Here's how the part is built. I have some questions about the finished solid (model axes, mm). Face numbers are marked on the shaded views. Coordinates: 2 decimals unless noted, no trailing zeros. Write each loop counter-clockwise with the first axis right and the second up, starting at its lowest first coordinate (ties: lowest second). Pieces come first, ordered by that corner, then holes.
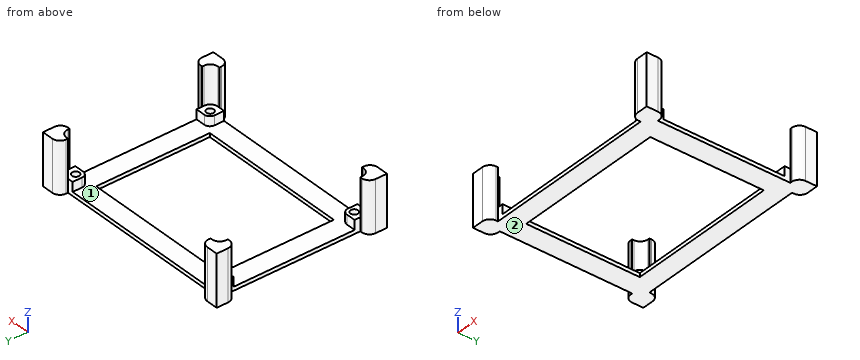
```python
from build123d import *

# Parameters (mm, degrees)
BOSS_EXTRUDE2_DEPTH = 27
SKETCH3_W           = 102
SKETCH3_H           = 80
CUT_EXTRUDE2_DEPTH  = 25
SKETCH4_W           = 8
SKETCH4_H           = 8
BOSS_EXTRUDE3_DEPTH = 5
SKETCH7_R           = 1.95
CUT_EXTRUDE3_DEPTH  = 3
FILLET2_R           = 3
FILLET3_R           = 4
SKETCH8_W           = 80
SKETCH8_H           = 60
CUT_EXTRUDE4_DEPTH  = 3


with BuildPart() as part:
    # Sketch1 → Boss-Extrude2 (new body)
    with BuildSketch(Plane.XY):
        Polygon((0, 75), (-5, 75), (-5, 85), (5, 85), (5, 80), (97, 80), (97, 85), (107, 85), (107, 75), (102, 75), (102, 5), (107, 5), (107, -5), (97, -5), (97, 0), (5, 0), (5, -5), (-5, -5), (-5, 5), (0, 5), align=None)
    extrude(amount=BOSS_EXTRUDE2_DEPTH)

    # Sketch3 → Cut-Extrude2 (cut)
    with BuildSketch(Plane.XY.offset(27)):
        with Locations((51, 40)):
            Rectangle(SKETCH3_W, SKETCH3_H)
    extrude(amount=-CUT_EXTRUDE2_DEPTH, mode=Mode.SUBTRACT)

    # Sketch4 → Boss-Extrude3 (add)
    with BuildSketch(Plane.XY.offset(2)):
        with Locations((4, 76)):
            Rectangle(SKETCH4_W, SKETCH4_H)
        with Locations((98, 76)):
            Rectangle(SKETCH4_W, SKETCH4_H)
        with Locations((98, 4)):
            Rectangle(SKETCH4_W, SKETCH4_H)
        with Locations((4, 4)):
            Rectangle(SKETCH4_W, SKETCH4_H)
    extrude(amount=BOSS_EXTRUDE3_DEPTH)

    # Sketch7 → Cut-Extrude3 (cut)
    with BuildSketch(Plane.XY.offset(7)):
        with Locations((4.5, 75.5)):
            Circle(SKETCH7_R)
        with Locations((97.5, 75.5)):
            Circle(SKETCH7_R)
        with Locations((97.5, 4.5)):
            Circle(SKETCH7_R)
        with Locations((4.5, 4.5)):
            Circle(SKETCH7_R)
    extrude(amount=-CUT_EXTRUDE3_DEPTH, mode=Mode.SUBTRACT)

    # Fillet2
    fillet2_edges = [part.edges().sort_by_distance(p)[0] for p in [
        (94, 72, 4.5),
        (94, 8, 4.5),
        (8, 8, 4.5),
        (8, 72, 4.5),
    ]]
    fillet(fillet2_edges, radius=FILLET2_R)

    # Fillet3
    fillet3_edges = [part.edges().sort_by_distance(p)[0] for p in [
        (102, 80, 17),
        (102, 0, 17),
        (0, 0, 17),
        (-5, 75, 13.5),
        (5, 85, 13.5),
        (97, 85, 13.5),
        (107, 75, 13.5),
        (107, 5, 13.5),
        (97, -5, 13.5),
        (5, -5, 13.5),
        (-5, 5, 13.5),
        (0, 80, 17),
    ]]
    fillet(fillet3_edges, radius=FILLET3_R)

    # Sketch8 → Cut-Extrude4 (cut, through all)
    with BuildSketch(Plane.XY.offset(2)):
        with Locations((51, 40)):
            Rectangle(SKETCH8_W, SKETCH8_H)
    extrude(amount=-CUT_EXTRUDE4_DEPTH, mode=Mode.SUBTRACT)


solid = part.part
```
1) Imagine slicing it at B-B on y = 32. Please give me the cut outline in (x, z), then the cut area to 3 significant figures.
Values follow:
outline: (0, 0) - (11, 0) - (11, 2) - (0, 2) - close; (91, 0) - (102, 0) - (102, 2) - (91, 2) - close
area: 44.0 mm2
2) We'd pull the mould along X, two halves only. Please class the marked faces 1 and 2: pulls with the +X half, pulls with the -X half, needs draft (parallel to the pull), parting line crosses it, or undercut.
Values follow:
face 1: undercut
face 2: needs draft
3) I need wall thicknesses on probe 1 along Y at (x, z) = (97.5, 6.05); probe 2 along X at (y, z) = (73.5, 4.75); probe 3 along X at (y, z) = (22, 1.25). Which ranges of each line are inside material? Lowest first, please.
Values follow:
probe 1: y = -2.94 to 2.55, 6.45 to 8, 72 to 73.55, 77.45 to 82.94
probe 2: x = 0 to 7.6, 94.4 to 102
probe 3: x = 0 to 11, 91 to 102
4) Will these pins go through, and if not, where does the flat tip stop? pin 1 (7.5 mm diameter, centred on x = 62.5, z = 3.5, fed in from -Y); pin 2 (1 mm diameter, centred on y = 45.5, z = 1.5, fed in from +X); pin 3 (2.5 mm diameter, centred on x = 97.5, y = 75.5, fed in from +Z); pin 4 (5 mm diameter, centred on x = 87.5, y = 48.5, fed in from +Z).
Values follow:
pin 1: stops at y = 0
pin 2: stops at x = 102
pin 3: stops at z = 4
pin 4: passes through
5) Imagine slicing it at C-C on z = 14.75. Count the separate pieces of the cut face and the enclosed holes in it, then the cut area to 3 significant figures.
Values follow:
separate pieces: 4
enclosed holes: 0
area: 286 mm2
6) Imagine slicing it at A-A on x = 47. Please give me the cut outline in (y, z).
Values follow:
outline: (0, 0) - (10, 0) - (10, 2) - (0, 2) - close; (70, 0) - (80, 0) - (80, 2) - (70, 2) - close
